from build123d import *

# Parameters (mm, degrees)
SKETCH2_R           = 5
BOSS_EXTRUDE2_DEPTH = 4
BOSS_EXTRUDE3_DEPTH = 65.921828


with BuildPart() as part:
    # Sketch2 → Boss-Extrude2 (new body)
    with BuildSketch(Plane(origin=(0, 0, 0), x_dir=(1, 0, 0), z_dir=(0, 1, 0))):
        with BuildLine():
            Line((0, 18), (18, 0))
            Line((18, 0), (96, 0))
            ThreePointArc((96, 0), (104.485281374, 3.514718626), (108, 12))
            Line((108, 12), (108, 26.188792937))
            Line((108, 26.188792937), (54, 64))
            Line((54, 64), (12, 64))
            ThreePointArc((12, 64), (3.514718626, 60.485281374), (0, 52))
            Line((0, 52), (0, 18))
        make_face()
        with Locations(Location((12, 52, 0), (0, 0, 270))):
            Circle(SKETCH2_R, mode=Mode.SUBTRACT)
        with Locations(Location((96, 12, 0), (0, 0, 270))):
            Circle(SKETCH2_R, mode=Mode.SUBTRACT)
    extrude(amount=BOSS_EXTRUDE2_DEPTH)

    # Sketch6 → Boss-Extrude3 (add)
    with BuildSketch(Plane(origin=(6.164380005, 0, 4.316345348), x_dir=(0.5735764363510455, 0, -0.8191520442889922), z_dir=(0.8191520442889922, 0, 0.5735764363510455))):
        with BuildLine():
            Line((91.356422356, 5.367444663), (94.832896583, 13.972020318))
            Line((94.832896583, 13.972020318), (91.124161165, 15.470446692))
            Line((91.124161165, 15.470446692), (87.647686938, 6.865871037))
            ThreePointArc((87.647686938, 6.865871037), (85.96136502, 4.783436896), (83.398858397, 4))
            Line((83.398858397, 4), (83.398858397, 0))
            ThreePointArc((83.398858397, 0), (88.198136634, 1.467286606), (91.356422356, 5.367444663))
        make_face()
    extrude(amount=BOSS_EXTRUDE3_DEPTH)


solid = part.part
Source: CAD feature listing. Evaluate the final solid. Frame: model axes, mm. A direction names the side the tool comes from. Round coordinates to 2 decimals unless told otherwise and drop trailing zeros. Order: outer loops, then holes, each group sorted by start corner. A loop starts at its lowest first (then second) coordinate and runs counter-clockwise, first axis right, second up. Notation, with made-up numbers: (31.5, 9) - (52.5, 9) arc R26 cw to (52.5, 26) - close; hole circle Ø11 at (-32, 5.5). An arc over 180 degrees is marked (long way). Use a Markdown table: item, result. Add a question column.
1. Section query A-A (y = 9). Return the cut outline in (x, z), then the cut area to 3 significant figures.
2. First-contact query: pin 1 (3 mm diameter, centred on x = 30.5, y = 3, fed in from +Z); pin 2 (19 mm diameter, centred on x = 53, z = -34, fed in from +Y); pin 3 (1.2 mm diameter, centred on y = 1.5, z = -21.5, fed in from +X); pin 4 (6 mm diameter, centred on x = 102.5, y = 11, fed in from +Z). Flat tips, straight axial feed; report the tip coordinate or a pass-through.
3. Mould query, pull axis Z, two halves, no side actions, for faces 6 (the cylindrical face through (91.12, 1.97, -13.08)), 7 (the flat face through (86.13, 14.71, -53.23)), 8 (the flat face through (9, 2, -9)), 9 (the cylindrical face through (15, 2, -56)). Classes: +Z half, -Z half, draft (parallel to the pull), parting line (faces both ways), or undercut.
4. Line query: probe 1 along Y at (x, z) = (19.5, -52); probe 2 along X at (y, z) = (1, -23); probe 3 along X at (y, z) = (3.05, -12). Output: solid intervals per line, ascending.
5. Set-up query: faces 1 (the flat face through (53, 4, -32)), 2 (the flat face through (86.17, 9.61, -53.28)), 3 (the flat face through (33, 2, -64)), 4 (the flat face through (53, 0, -32)), 5 (the flat face through (108, 2, -19)). Return all of +Z, -Z, +X, -X, +Y, -Y with unobstructed straight access to the full face (end or side cutting, diameter ignored); none if empty.
Derived:
| question | item | result |
|---|---|---|
| 1 | outline | (56.93, -68.19) - (59.41, -71.72) - (113.41, -33.91) - (110.93, -30.38) - close |
| 1 | area | 284 mm2 |
| 2 | pin 1 | z = 0 |
| 2 | pin 2 | y = 4 |
| 2 | pin 3 | x = 108 |
| 2 | pin 4 | z = -34.7 |
| 3 | face 6 | undercut |
| 3 | face 7 | -Z half |
| 3 | face 8 | +Z half |
| 3 | face 9 | undercut |
| 4 | probe 1 | 0 to 4 |
| 4 | probe 2 | 0 to 108 |
| 4 | probe 3 | 6 to 91, 101 to 108 |
| 5 | face 1 | +Z, -X, +Y |
| 5 | face 2 | -Z, +X, -Y |
| 5 | face 3 | -Z, -X, +Y, -Y |
| 5 | face 4 | +Z, -Z, +X, -X, -Y |
| 5 | face 5 | +Z, +X, +Y, -Y |
